Autodesk Inventor part; units mm, degrees
ref_plane "YZ Plane" through (0, 0, 0) normal (1, 0, 0) x (0, 1, 0)
ref_plane "XZ Plane" through (0, 0, 0) normal (0, 1, 0) x (-1, 0, 0)
ref_plane "XY Plane" through (0, 0, 0) normal (0, 0, 1) x (1, 0, 0)
sketch "Sketch7" plane through (0, 0, 0) normal (0, 0, 1) x (1, 0, 0)
  circle A0 centre (0, 0) radius 302.5
  line L0 (0, 0) -> (500, 0) construction
  line L1 (0, 0) -> (433.0127, -250) construction
  line L2 (0, 0) -> (500, 0) construction
  line L3 (0, 0) -> (-433.0127, -250) construction
  line L4 (0, 0) -> (500, 0) construction
  circle A1 centre (0, 224) radius 40.5
  circle A2 centre (-193.9897, -112) radius 40.5
  circle A3 centre (193.9897, -112) radius 40.5
  circle A4 centre (0, -240) radius 37.5
  circle A5 centre (0, 0) radius 120
  circle A6 centre (0, 0) radius 293.8 construction
  line L5 (-461.9398, -191.3417) -> (461.9398, 191.3417) construction
  line L6 (0, 0) -> (191.3417, 461.9398) construction
  line L7 (0, 0) -> (500, 0) construction
  circle A7 centre (0, 293.8) radius 2.5
  circle A8 centre (0, 293.8) radius 4.225 construction
  circle A9 centre (0, 293.8) radius 5 construction
  circle A10 centre (271.4358, 112.4324) radius 5 construction
  circle A11 centre (271.4358, 112.4324) radius 2.5
  line L8 (275.8097, 114.2441) -> (275.1918, 109.5504) construction
  line L9 (275.1918, 109.5504) -> (270.8179, 107.7386) construction
  line L10 (270.8179, 107.7386) -> (267.0619, 110.6207) construction
  line L11 (267.0619, 110.6207) -> (267.6799, 115.3144) construction
  line L12 (267.6799, 115.3144) -> (272.0538, 117.1262) construction
  line L13 (272.0538, 117.1262) -> (275.8097, 114.2441) construction
  circle A12 centre (112.4324, 271.4358) radius 5 construction
  circle A13 centre (112.4324, 271.4358) radius 2.5
  line L14 (114.2441, 275.8097) -> (117.1262, 272.0538) construction
  line L15 (117.1262, 272.0538) -> (115.3144, 267.6799) construction
  line L16 (115.3144, 267.6799) -> (110.6207, 267.0619) construction
  line L17 (110.6207, 267.0619) -> (107.7386, 270.8179) construction
  line L18 (107.7386, 270.8179) -> (109.5504, 275.1918) construction
  line L19 (109.5504, 275.1918) -> (114.2441, 275.8097) construction
  circle A14 centre (-271.4358, -112.4324) radius 5 construction
  circle A15 centre (-271.4358, -112.4324) radius 2.5
  line L20 (-275.8097, -114.2441) -> (-275.1918, -109.5504) construction
  line L21 (-275.1918, -109.5504) -> (-270.8179, -107.7386) construction
  line L22 (-270.8179, -107.7386) -> (-267.0619, -110.6207) construction
  line L23 (-267.0619, -110.6207) -> (-267.6799, -115.3144) construction
  line L24 (-267.6799, -115.3144) -> (-272.0538, -117.1262) construction
  line L25 (-272.0538, -117.1262) -> (-275.8097, -114.2441) construction
  circle A16 centre (-207.748, 207.748) radius 2.5
  circle A17 centre (-207.748, 207.748) radius 4.225 construction
  circle A18 centre (-207.748, 207.748) radius 5 construction
  circle A19 centre (-293.8, 0) radius 2.5
  circle A20 centre (-293.8, 0) radius 4.225 construction
  circle A21 centre (-293.8, 0) radius 5 construction
  circle A22 centre (-207.748, -207.748) radius 2.5
  circle A23 centre (-207.748, -207.748) radius 4.225 construction
  circle A24 centre (-207.748, -207.748) radius 5 construction
  circle A25 centre (0, -293.8) radius 2.5
  circle A26 centre (0, -293.8) radius 4.225 construction
  circle A27 centre (0, -293.8) radius 5 construction
  circle A28 centre (207.748, -207.748) radius 2.5
  circle A29 centre (207.748, -207.748) radius 4.225 construction
  circle A30 centre (207.748, -207.748) radius 5 construction
  circle A31 centre (293.8, 0) radius 2.5
  circle A32 centre (293.8, 0) radius 4.225 construction
  circle A33 centre (293.8, 0) radius 5 construction
  circle A34 centre (207.748, 207.748) radius 2.5
  circle A35 centre (207.748, 207.748) radius 4.225 construction
  circle A36 centre (207.748, 207.748) radius 5 construction
  dimension "d26" = 605
  dimension "d29" = 500
  dimension "d30" = 30
  dimension "d31" = 500
  dimension "d32" = 150
  dimension "d34" = 81
  dimension "d35" = 224
  dimension "d38" = 360
  dimension "d40" = 75
  dimension "d41" = 240
  dimension "d42" = 240
  dimension "d79" = 587.6
  dimension "d80" = 1000
  dimension "d82" = 500
  dimension "d83" = 67.5
  dimension "d84" = 5
  dimension "d85" = 8.45
  dimension "d86" = 10
  dimension "d87" = 10
  dimension "d88" = 5
  dimension "d89" = 8.2
  dimension "d90" = 10
  dimension "d91" = 5
  dimension "d92" = 8.2
  dimension "d93" = 10
  dimension "d94" = 5
  dimension "d95" = 8.2
  dimension "d98" = 360
extrude "Extrusion7" add sketch "Sketch7" against normal blind 12.2 contours A0 | A1 | A2 | A3 | A4 | A5 | A7 | A11 | A13 | A15 | A16 | A19 | A22 | A25 | A28 | A31 | A34
extrude "Extrusion8" add sketch "Sketch7" along normal blind 30.25 contours A1 | A2 | A3
extrude "Extrusion9" add sketch "Sketch7" along normal blind 10.7 contours A5
extrude "Extrusion10" add sketch "Sketch7" along normal blind 15.25 contours A4
extrude "Extrusion11" cut sketch "Sketch7" against normal blind 12.2 contours A7 | A11 | A13 | A15 | A16 | A19 | A22 | A25 | A28 | A31 | A34
fillet "Fillet4" radius 1 4 edges at (-120, 0, 10.7) (-120, 0, 0) (-302.5, 0, 0) (-302.5, 0, -12.2)
properties part number "proteox_tube_bottom" material "Stainless Steel"
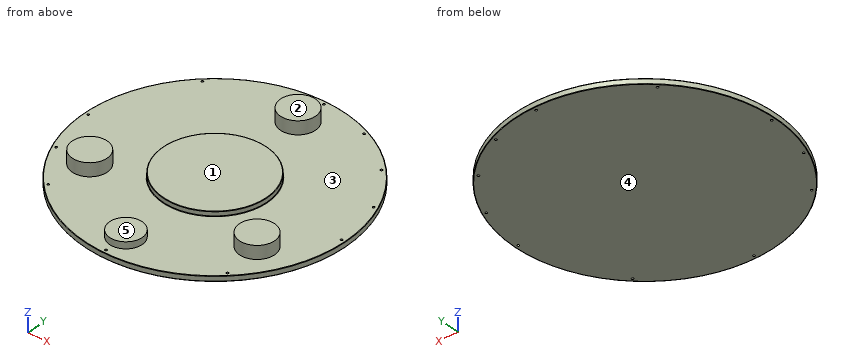
Check sheet for the modelled part. Datum: model origin and axes. Units: mm. Face numbers are marked on the shaded views. A direction names the side the tool comes from. Round coordinates to 2 decimals unless told otherwise and drop trailing zeros. Order: outer loops, then holes, each group sorted by start corner. A loop starts at its lowest first (then second) coordinate and runs counter-clockwise, first axis right, second up. Notation, with made-up numbers: (87, 55.25) - (98, 55.25) arc R8 ccw to (98, 67.25) - close; hole circle Ø7 at (61.25, -19.75). An arc over 180 degrees is marked (long way). Write item = value, one per line.
Q1. Tool access check on the marked faces 3, 4 and 5. Record the directions out of +Z, -Z, +X, -X, +Y, -Y that give a thin tool (end or side, any length) a straight path to the whole face; none if there is none.
Computed:
face_3 = +Z
face_4 = -Z, +X, -X, +Y, -Y
face_5 = +Z, +X, -X, -Y
Q2. Draft check along Y on the marked faces 1 and 2. Enter one of: pulls with the +Y half, pulls with the -Y half, needs draft (parallel to the pull), parting line crosses it, or undercut.
Computed:
face_1 = undercut
face_2 = needs draft
Q3. Thickness scan on line 1 along Y through (x, z) = (0, -2); line 2 along Y through (x, z) = (2, 9.5); line 3 along Z through (x, y) = (-105, -77). Record the ranges inside material, lowest first.
Computed:
line_1 = -302.5 to -296.3, -291.3 to 291.3, 296.3 to 302.5
line_2 = -277.45 to -202.55, -119.98 to 119.98, 183.55 to 264.45
line_3 = -12.2 to 0
Q4. Go/stop test with flat-tipped pins: pin 1 (6.5 mm diameter, centred on x = -207.748, y = -207.748, fed in from +Z); pin 2 (10 mm diameter, centred on y = -234, z = 1, fed in from -X); pin 3 (6.5 mm diameter, centred on x = 0, y = -293.8, fed in from -Z); pin 4 (6 mm diameter, centred on y = -85.5, z = 7, fed in from -X). Record where each tip stops, or that it passes through.
Computed:
pin_1 = 0
pin_2 = -197.23
pin_3 = -12.2
pin_4 = -226.97
Q5. Section check A-A (z = 22.5). Record the boundary of the cut face in (x, y).
Computed:
outline = circle Ø81 at (-193.99, -112); circle Ø81 at (0, 224); circle Ø81 at (193.99, -112)
